Source: CAD feature listing. Evaluate the final solid. Frame: model axes, mm. Face numbers are marked on the shaded views. A direction names the side the tool comes from. Give positions to 0.01 mm unless a question says otherwise; leave off trailing zeros. Order: outer loops, then holes, each group sorted by start corner. A loop starts at its lowest first (then second) coordinate and runs counter-clockwise, first axis right, second up. Notation, with made-up numbers: (89, -14.5) - (102, -14.5) arc R6 ccw to (102, -10.5) - close; hole circle Ø9 at (89.5, 2). An arc over 180 degrees is marked (long way). One line per item, written item: value. Start each with the question number.
from build123d import *

# Parameters (mm, degrees)
CUT_EXTRUDE1_DEPTH = 25
CUT_EXTRUDE2_DEPTH = 22
SKETCH4_R          = 1.6
CUT_EXTRUDE3_DEPTH = 53.981423697
FILLET3_R          = 0.5
FILLET6_R          = 2
FILLET7_R          = 1


with BuildPart() as part:
    # Sketch1 → Revolve1 (revolve)
    with BuildSketch(Plane.XY, mode=Mode.PRIVATE) as revolve1_sk:
        with BuildLine():
            Line((-28.125, 0), (-28.125, 3))
            Line((-28.125, 3), (-16.125, 3))
            ThreePointArc((-16.125, 3), (-14.357841488, 20.846568298), (-9.125, 38))
            Line((-9.125, 38), (-7.125, 38))
            Line((-7.125, 38), (-7.125, 0))
            Line((-7.125, 0), (-28.125, 0))
        make_face()
    revolve(revolve1_sk.sketch.rotate(Axis((0, 0, 0), (0, 1, 0)), 270), axis=Axis((0, 0, 0), (0, 1, 0)))

    # Sketch2 → Cut-Extrude1 (cut)
    with BuildSketch(Plane.XZ):
        Polygon((0, 12.817175976), (-11.1, 6.408587988), (-11.1, -6.408587988), (0, -12.817175976), (11.1, -6.408587988), (11.1, 6.408587988), align=None)
    extrude(amount=-CUT_EXTRUDE1_DEPTH, mode=Mode.SUBTRACT)

    # Sketch3 → Cut-Extrude2 (cut)
    with BuildSketch(Plane(origin=(0, 3, 0), x_dir=(1, 0, 0), z_dir=(0, 1, 0))):
        with BuildLine():
            ThreePointArc((17.421699831, -5), (12.816310409, -12.816310409), (5, -17.421699831))
            Line((5, -17.421699831), (5, -27.676987282))
            ThreePointArc((5, -27.676987282), (19.887378221, -19.887378221), (27.676987282, -5))
            Line((27.676987282, -5), (17.421699831, -5))
        make_face()
        with BuildLine():
            Line((-5, -27.676987282), (-5, -17.421699831))
            ThreePointArc((-5, -17.421699831), (-12.816310409, -12.816310409), (-17.421699831, -5))
            Line((-17.421699831, -5), (-27.676987282, -5))
            ThreePointArc((-27.676987282, -5), (-19.887378221, -19.887378221), (-5, -27.676987282))
        make_face()
        with BuildLine():
            Line((-27.676987282, 5), (-17.421699831, 5))
            ThreePointArc((-17.421699831, 5), (-12.816310409, 12.816310409), (-5, 17.421699831))
            Line((-5, 17.421699831), (-5, 27.676987282))
            ThreePointArc((-5, 27.676987282), (-19.887378221, 19.887378221), (-27.676987282, 5))
        make_face()
        with BuildLine():
            ThreePointArc((5, 17.421699831), (12.816310409, 12.816310409), (17.421699831, 5))
            Line((17.421699831, 5), (27.676987282, 5))
            ThreePointArc((27.676987282, 5), (19.887378221, 19.887378221), (5, 27.676987282))
            Line((5, 27.676987282), (5, 17.421699831))
        make_face()
    extrude(amount=-CUT_EXTRUDE2_DEPTH, mode=Mode.SUBTRACT)

    # Sketch4 → Cut-Extrude3 (cut, through all)
    with BuildSketch(Plane(origin=(0, 3, 0), x_dir=(1, 0, 0), z_dir=(0, 1, 0))):
        with Locations(Location((23.125, 0, 0), (0, 0, 270))):
            Circle(SKETCH4_R)
        with Locations(Location((0, -23.125, 0), (0, 0, 270))):
            Circle(SKETCH4_R)
        with Locations(Location((-23.125, 0, 0), (0, 0, 270))):
            Circle(SKETCH4_R)
        with Locations(Location((0, 23.125, 0), (0, 0, 270))):
            Circle(SKETCH4_R)
    extrude(amount=-CUT_EXTRUDE3_DEPTH, mode=Mode.SUBTRACT)

    # Fillet3
    fillet3_edges = [part.edges().sort_by_distance(p)[0] for p in [
        (5.55, 25, 9.612881982),
        (11.1, 25, 0),
        (5.55, 25, -9.612881982),
        (-5.55, 25, -9.612881982),
        (-11.1, 25, 0),
        (-5.55, 25, 9.612881982),
        (0, 25, 7.125),
        (0, 38, 7.125),
    ]]
    fillet(fillet3_edges, radius=FILLET3_R)

    # Fillet6
    fillet6_edges = [part.edges().sort_by_distance(p)[0] for p in [
        (-17.421699831, 1.5, 5),
        (-5, 1.5, 17.421699831),
        (-5, 1.5, 27.676987282),
        (-27.676987282, 1.5, 5),
        (5, 1.5, 17.421699831),
        (17.421699831, 1.5, 5),
        (27.676987282, 1.5, 5),
        (5, 1.5, 27.676987282),
        (17.421699831, 1.5, -5),
        (5, 1.5, -17.421699831),
        (5, 1.5, -27.676987282),
        (27.676987282, 1.5, -5),
        (-5, 1.5, -17.421699831),
        (-17.421699831, 1.5, -5),
        (-27.676987282, 1.5, -5),
        (-5, 1.5, -27.676987282),
    ]]
    fillet(fillet6_edges, radius=FILLET6_R)

    # Fillet7
    fillet7_edges = [part.edges().sort_by_distance(p)[0] for p in [
        (0, 3, 16.125),
    ]]
    fillet(fillet7_edges, radius=FILLET7_R)


solid = part.part
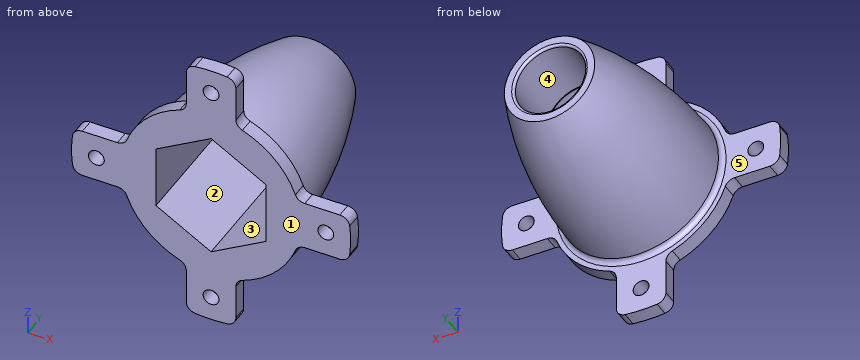
1. Contact query for flat-ended pins moving along their axis: pin 1 Ø2.5 at (x, y) = (-22, 1.5) entering from -Z; pin 2 Ø8 at (y, z) = (24, -8) entering from -X; pin 3 Ø8 at (x, y) = (6.5, 28) entering from -Z. Output: stop coordinate, or through.
2. Set-up query: the marked faces 3, 4 and 5. Return all of +Z, -Z, +X, -X, +Y, -Y with unobstructed straight access to the full face (end or side cutting, diameter ignored); none if empty.
3. Draft query along X for the marked faces 1 and 2. Return one class per face: pulls with the +X half, pulls with the -X half, needs draft (parallel to the pull), parting line crosses it, or undercut.
4. Ray query, L1, parallel to X at y = 1.3, z = 0 (3 decimals); L2, parallel to Z at x = 4, y = 4; L3, parallel to Z at x = 11, y = 16. Return the intervals inside material, ascending.
5. Section A-A on z = 0. Count the separate pieces of the cut face and the enclosed holes in it, then the cut area to 3 significant figures.
6. Section B-B on x = 20. Return the cut outline in (y, z), then the cut area to 3 significant figures.
Data:
1. pin 1: stops at z = -5
1. pin 2: stops at x = -13.37
1. pin 3: stops at z = -12.87
2. face 3: -Y
2. face 4: +Y, -Y
2. face 5: +Y
3. face 1: needs draft
3. face 2: undercut
4. L1: x = -28.125 to -24.725, -21.525 to -11.1, 11.1 to 21.525, 24.725 to 28.125
4. L2: z = -15.62 to -10.51, 10.51 to 15.62
4. L3: z = -10.48 to -6.47, 6.47 to 10.48
5. separate pieces: 4
5. enclosed holes: 0
5. area: 378 mm2
6. outline: (0, -5) - (3, -5) - (3, 5) - (0, 5) - close
6. area: 30.0 mm2
